Source: CAD feature listing. Evaluate the final solid. Frame: model axes, mm. Face numbers are marked on the shaded views. A direction names the side the tool comes from. Give positions to 0.01 mm unless a question says otherwise; leave off trailing zeros. Order: outer loops, then holes, each group sorted by start corner. A loop starts at its lowest first (then second) coordinate and runs counter-clockwise, first axis right, second up.
1) Section A-A, the plane z = -28. Return loops of the section in (x, y).
2) Material intervals for line 1 (Z direction, x = 2.25, y = 5.25); line 2 (Z direction, x = 1, y = 3.5); line 3 (Z direction, x = -0.25, y = 1.25), sorted ascending.
3) Access query for the marked faces 1 and 2. Directions: +Z, -Z, +X, -X, +Y, -Y. A direction counts if a zero-diameter tool reaches every point of the face in a straight line with its end or side. Return the directions, or none.
4) First-contact query: P1, Ø1.9, axis at x = 3, z = 3, coming from the +Y side; P2, Ø1.2, axis at y = 2.5, z = 2.5, coming from the +X side; P3, Ø1.2, axis at y = -3, z = 2, coming from the -X side; P4, Ø1.5, axis at x = -6.5, z = -16.5, coming from the +Y side. Flat tips, straight axial feed; report the tip coordinate or a pass-through.
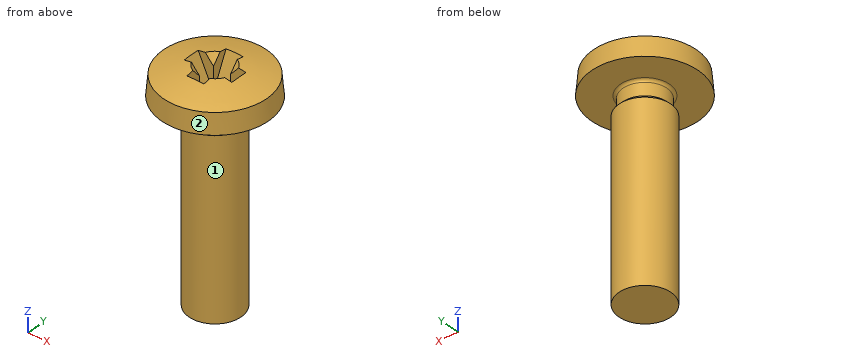
Autodesk Inventor part; units mm, degrees
ref_plane "MSC_PF1" through (0, 0, 0) normal (1, 0, 0) x (0, 1, 0)
ref_plane "MSC_PT1" through (0, 0, 0) normal (0, 0, -1) x (-1, 0, 0)
ref_plane "YZ Plane" through (0, 0, 0) normal (1, 0, 0) x (0, 1, 0)
sketch "Эскиз2" plane through (0, 0, 0) normal (0, 0, 1) x (1, 0, 0)
  circle A0 centre (0, 0) radius 3.375
  dimension "d3" = 6.75
extrude "Выдавливание1" add sketch "Эскиз2" against normal blind 2.34
sketch "Эскиз3" plane through (0, 0, -2.34) normal (0, 0, -1) x (-1, 0, 0)
  circle A0 centre (0, 0) radius 4
  circle A1 centre (0, 0) radius 3.375 construction
  dimension "d28" = 360
  dimension "d9" = 8
extrude "Выдавливание2" add sketch "Эскиз3" along normal blind 27.66
chamfer "Фаска1" distance 0.625 distance2 0.625 1 edges at (4, 0, -2.34) measured on face at (-3.7202, -0.5883, -2.34)
sketch "Эскиз4" plane through (0, 0, 0) normal (0, 0, 1) x (1, 0, 0)
  circle A0 centre (0, 0) radius 8.2
  circle A1 centre (0, 0) radius 3.375 construction
  dimension "d15" = 16.4
extrude "Выдавливание3" add sketch "Эскиз4" along normal blind 3.1
fillet "Сопряжение1" radius 0.4 1 edges at (-3.375, 0, 0)
sketch "Эскиз5" plane through (0, 0, 0) normal (0, 1, 0) x (-1, 0, 0)
  line L0 (8.2, 3.1) -> (8.2, 0)
  line L1 (7.9288, 3.1) -> (8.2, 3.1)
  line L2 (8.2, 0) -> (7.9288, 3.1)
  line L3 (-8.2, 3.1) -> (8.2, 3.1) construction
  line L4 (-8.2, 0) -> (8.2, 0) construction
  line L5 (0, -0.62) -> (0, 3.72)
  line L6 (11.48, 0) -> (-11.48, 0)
  dimension "d20" = 5
  dimension "d56" = 8.2
  dimension "d57" = 3.1
revolve "Вращение1" cut sketch "Эскиз5" angle 360 about axis through (0, 0, -10) along (0, 0, 1)
sketch "Эскиз6" plane through (0, 0, 0) normal (0, 1, 0) x (-1, 0, 0)
  line L0 (0, 4.8) -> (0, 3.1)
  arc A0 (7.9288, 3.1) -> (0, 4.8) centre (-2.8592, -27.8751) ccw
  line L1 (0, 3.1) -> (7.9288, 3.1)
  line L2 (7.9288, 3.1) -> (-7.9288, 3.1) construction
  line L3 (0, -4.4495) -> (0, 0.4495)
  line L4 (0, -34.4594) -> (0, 11.6302)
  line L5 (11.1636, 0) -> (-11.1108, 0)
  dimension "d58" = 1.7
  dimension "d59" = 7.9288
  dimension "d60" = 0
  dimension "d62" = 32.8
revolve "Вращение2" add sketch "Эскиз6" angle 360 about axis through (0, 0, -4.4495) along (0, 0, 1)
sketch "Эскиз7" plane through (0, 0, 0) normal (0, 1, 0) x (-1, 0, 0)
  line L0 (3.9, 4.8) -> (-3.9, 4.8)
  line L1 (1.8669, 0.44) -> (3.9, 4.8)
  line L2 (-1.8669, 0.44) -> (1.8669, 0.44)
  line L3 (-3.9, 4.8) -> (-1.8669, 0.44)
  line L4 (0, -0.432) -> (0, 5.672)
  line L5 (5.46, 0) -> (-5.46, 0)
  dimension "d32" = 4.36
  dimension "d34" = 65
  dimension "d36" = 65
  dimension "d63" = 3.9
  dimension "d64" = 4.8
  dimension "d65" = 7.8
extrude "Выдавливание4" cut sketch "Эскиз7" against normal mid plane 2.6
sketch "Эскиз8" plane through (0, 0, 0) normal (1, 0, 0) x (0, 1, 0)
  line L0 (-1.8669, 0.44) -> (-3.9, 4.8)
  line L1 (1.8669, 0.44) -> (-1.8669, 0.44)
  line L2 (3.9, 4.8) -> (1.8669, 0.44)
  line L3 (-3.9, 4.8) -> (3.9, 4.8)
  line L4 (0, -0.432) -> (0, 5.672)
  line L5 (-5.46, 0) -> (5.46, 0)
  dimension "d40" = 65
  dimension "d42" = 65
  dimension "d44" = 4.36
  dimension "d66" = 7.8
  dimension "d67" = 4.8
  dimension "d69" = 3.9
extrude "Выдавливание5" cut sketch "Эскиз8" along normal mid plane 2.6
sketch "Эскиз9" plane through (0, 0, 0) normal (0, 1, 0) x (-1, 0, 0)
  line L0 (0, 4.8) -> (0, 0.44)
  line L1 (3.12, 4.8) -> (0, 4.8)
  line L2 (0, 0.44) -> (3.12, 4.8)
  line L3 (-8.2, 0) -> (8.2, 0) construction
  line L4 (0, -0.96) -> (0, 5.76)
  line L5 (11.48, 0) -> (-11.48, 0)
  dimension "d50" = 4.36
  dimension "d52" = 4.36
  dimension "d54" = 3.12
  dimension "d70" = 0
  dimension "d71" = 4.8
revolve "Вращение3" cut sketch "Эскиз9" angle 360 about axis through (0, 0, -10) along (0, 0, 1)
thread "Резьба1"
ref_plane "MSC_PF1" through (0, 0, 0) normal (1, 0, 0) x (0, 1, 0)
ref_plane "MSC_PT1" through (0, 0, 0) normal (0, 0, -1) x (-1, 0, 0)
equation "\"d4\" = -b + NLG"
equation "\"d9\" = NND"
equation "\"d10\" = b"
equation "\"d12\" = -0.5 * msp_ds + 0.5 * NND"
equation "\"d13\" = 0.5 * NND - 0.5 * msp_ds"
equation "\"d15\" = Dk"
equation "\"d16\" = ParK"
equation "\"d18\" = r"
equation "\"d32\" = q"
equation "\"d63\" = 0.5 * M"
equation "\"d64\" = ParK + ParF"
equation "\"d65\" = M"
equation "\"d37\" = 2 * msp_s"
equation "\"d44\" = q"
equation "\"d66\" = M"
equation "\"d67\" = ParK + ParF"
equation "\"d69\" = 0.5 * M"
equation "\"d47\" = 2 * msp_s"
equation "\"d3\" = msp_ds"
equation "\"d56\" = 0.5 * Dk"
equation "\"d57\" = ParK"
equation "\"d58\" = ParF"
equation "\"d59\" = 0.5 * Dk - msp_v"
equation "\"d62\" = 2 * Dk"
equation "\"d50\" = q"
equation "\"d52\" = q"
equation "\"d54\" = msp_rr"
equation "\"d71\" = ParK + ParF"
equation "\"PTC\" = 1.25"
equation "\"NLG\" = 30"
equation "\"Dk\" = 16.4"
equation "\"ParK\" = 3.1"
equation "\"NND\" = 8"
equation "\"M\" = 7.8"
equation "\"q\" = 4.36"
equation "\"r\" = 0.4"
equation "\"msp_ds\" = NND - PTC"
equation "\"b\" = 27.66"
equation "\"msp_x\" = 1.25 * PTC"
equation "\"msp_s\" = 0.166667 * M"
equation "\"msp_rr\" = 0.4 * M"
equation "\"ParF\" = 1.7"
equation "\"msp_v\" = 0.0874887 * ParK"
equation "\"THREADDIA\" = NND"
properties part number "JIS B 1111 - M8x30" material "Сталь, мягкая"
From the geometry:
1. outline: circle Ø8 at (0, 0)
2. line 1: z = 0 to 3.79
2. line 2: z = -30 to -2.6, -0.02 to 3.94
2. line 3: z = -30 to 0.44
3. face 1: -Z
3. face 2: +Z
4. P1: stops at y = 7.68
4. P2: stops at x = 7.76
4. P3: stops at x = -7.67
4. P4: passes through
